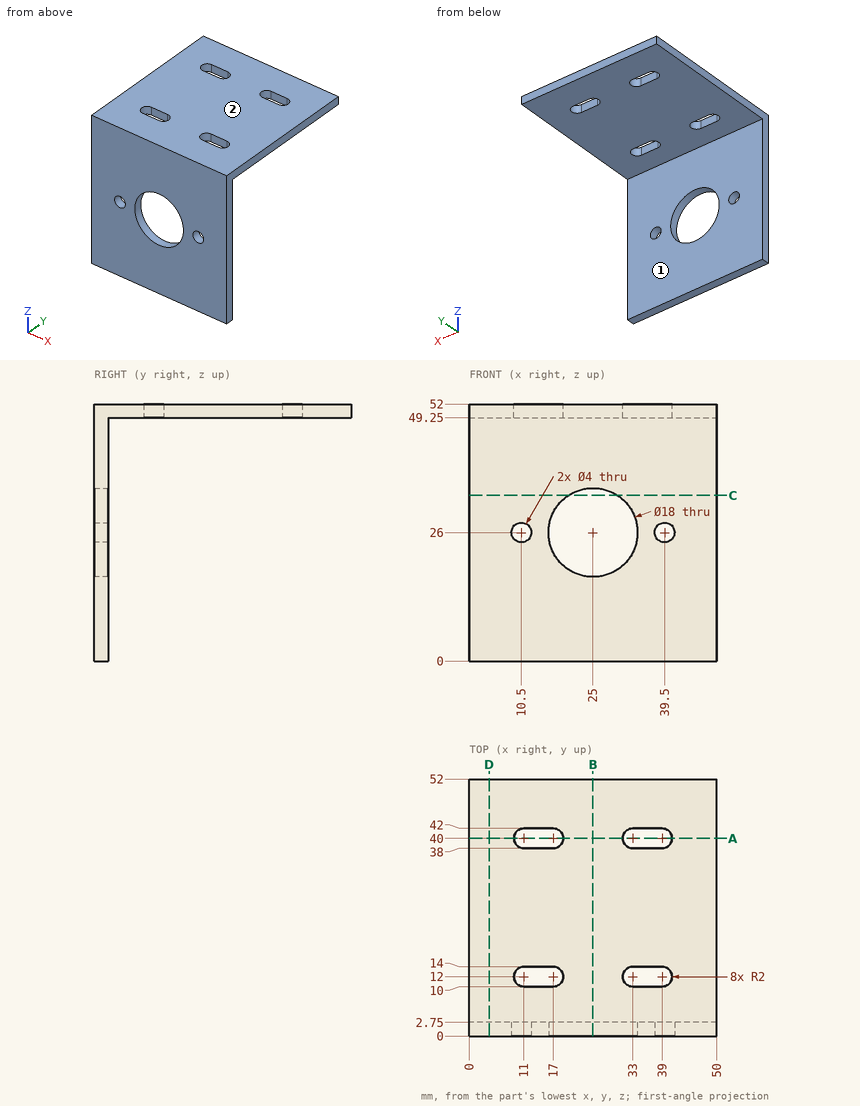
Here's the drawing with two shaded views (mm, measured from the low corner). I have some questions. A direction names the side the tool comes from. Give positions to 0.01 mm unless a question says otherwise; leave off trailing zeros. Write each loop counter-clockwise with the first axis right and the second up, starting at its lowest first coordinate (ties: lowest second). Pieces come first, ordered by that corner, then holes. Notation, with made-up numbers: (-18.75, -38.75) -> (31.25, -38.75) arc R7 ccw to (31.25, -27.75) -> close; hole circle Ø3 at (70.25, -1.5). An arc over 180 degrees is marked (long way). One line per item, written item: value.
Q1. Imagine slicing it at A-A on y = 40. Please give me the cut outline in (x, z).
Results found:
outline: (0, 49.25) -> (9, 49.25) -> (9, 52) -> (0, 52) -> close; (19, 49.25) -> (31, 49.25) -> (31, 52) -> (19, 52) -> close; (41, 49.25) -> (50, 49.25) -> (50, 52) -> (41, 52) -> close
Q2. Which directions (+Z, -Z, +X, -X, +Y, -Y) give clear straight access to the entire face, cutting with the end or side of a thin tool? Please do the marked faces 1 and 2.
Results found:
face 1: -Z, +X, -X, +Y
face 2: +Z, +X, -X, +Y, -Y
Q3. For P1, Ø3, axis at x = 39.5, z = 26, coming from the +Y side; P2, Ø5, axis at x = 10.5, z = 26, coming from the +Y side; P3, Ø2, axis at x = 11, y = 19, coming from the -Z side, each with a flat end and sliding along its axis, tell me the tip position at first contact or that it passes through.
Results found:
P1: passes through
P2: stops at y = 2.75
P3: stops at z = 49.25
Q4. Imagine slicing it at D-D on x = 4. Please give me the cut outline in (y, z), and give its area (3 significant figures).
Results found:
outline: (0, 0) -> (2.75, 0) -> (2.75, 49.25) -> (52, 49.25) -> (52, 52) -> (0, 52) -> close
area: 278 mm^2
Q5. Imagine slicing it at C-C on z = 33.5. Please give me the cut outline in (x, y), and give its area (3 significant figures).
Results found:
outline: (0, 0) -> (20.03, 0) -> (20.03, 2.75) -> (0, 2.75) -> close; (29.97, 0) -> (50, 0) -> (50, 2.75) -> (29.97, 2.75) -> close
area: 110 mm^2
Q6. Please list where these lines run through material, in increasing order: line 1 (X direction, y = 1, z = 26); line 2 (Y direction, x = 22, z = 11); line 3 (Z direction, x = 3, y = 41). Write a range as [from, to].
Results found:
line 1: x = [0, 8.5], [12.5, 16], [34, 37.5], [41.5, 50]
line 2: y = [0, 2.75]
line 3: z = [49.25, 52]
Q7. Imagine slicing it at B-B on x = 25. Please give me the cut outline in (y, z).
Results found:
outline: (0, 0) -> (2.75, 0) -> (2.75, 17) -> (0, 17) -> close; (0, 35) -> (2.75, 35) -> (2.75, 49.25) -> (52, 49.25) -> (52, 52) -> (0, 52) -> close
